```python
from build123d import *

# Parameters (mm, degrees)
F0_W      = 40
F0_H      = 20
F1_DEPTH  = 25
F2_W      = 10
F2_H      = 40
F3_DEPTH  = 25
F4_W      = 10
F4_H      = 2.6823076606
F5_DEPTH  = 50
F7_DEPTH  = 50
F8_R      = 14.99999
F9_F1_R   = 14.9999
F10_W     = 10
F10_H     = 10
F11_DEPTH = 100


# Not quite as in the source:
# - a fillet or chamfer is up to 0.001 mm smaller than in the source, because OpenCascade refuses the exact size


with BuildPart() as f1:
    # F0 (on Right) → F1 (new body)
    with BuildSketch(Plane.YZ):
        with Locations((20, 10)):
            Rectangle(F0_W, F0_H)
    extrude(amount=F1_DEPTH)

    # F2 (on face) → F3 (join)
    with BuildSketch(Plane.XY.offset(20)):
        with Locations((5, 20)):
            Rectangle(F2_W, F2_H)
    extrude(amount=F3_DEPTH)

    # F4 (on face) → F5 (cut)
    with BuildSketch(Plane.YZ.offset(10)):
        with BuildLine():
            Line((15, 45), (15, 35))
            ThreePointArc((15, 35), (20, 30), (25, 35))
            Line((25, 35), (25, 45))
            Line((25, 45), (15, 45))
        make_face()
        with Locations((20, 46.3411538303)):
            Rectangle(F4_W, F4_H)
    extrude(amount=-F5_DEPTH, mode=Mode.SUBTRACT)

    # F6 (on face) → F7 (cut)
    with BuildSketch(Plane.XY.offset(20)):
        with BuildLine():
            Line((25, 22.5), (15, 22.5))
            ThreePointArc((15, 22.5), (12.5, 20), (15, 17.5))
            Line((15, 17.5), (25, 17.5))
            Line((25, 17.5), (25, 22.5))
        make_face()
    extrude(amount=-F7_DEPTH, mode=Mode.SUBTRACT)

    # F8 (radius 15 in the source; OpenCascade refuses exactly that, so slightly less here)
    f8_edges = [f1.edges().sort_by_distance(p)[0] for p in [
        (5, 40, 45),
        (5, 0, 45),
    ]]
    fillet(f8_edges, radius=F8_R)

    # F9: fillet of radius 15 on 2 edges, made by hand

    # F9_f1 (radius 15 in the source; OpenCascade refuses exactly that, so slightly less here)
    f9_f1_edges = [f1.edges().sort_by_distance(p)[0] for p in [
        (25, 8.75, 20),
    ]]
    fillet(f9_f1_edges, radius=F9_F1_R)

    # F10 (on face) → F11 (cut)
    with BuildSketch(Plane(origin=(0, 40, 0), x_dir=(-1, 0, 0), z_dir=(0, 1, 0))):
        with Locations((-15, 5)):
            Rectangle(F10_W, F10_H)
    extrude(amount=-F11_DEPTH, mode=Mode.SUBTRACT)


solid = f1.part
```
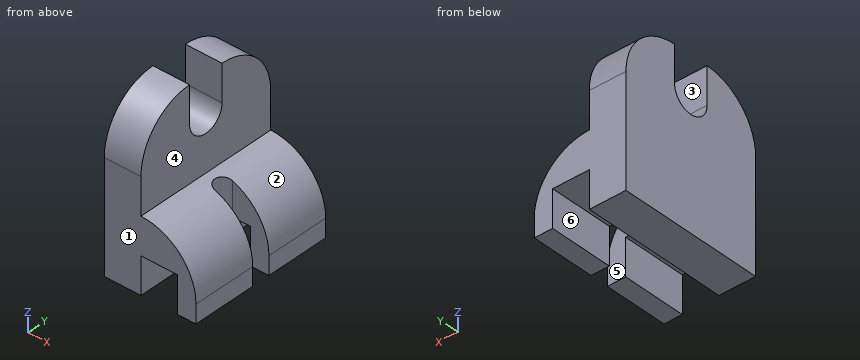
Source: CAD feature listing. Evaluate the final solid. Frame: model axes, mm. Face numbers are marked on the shaded views. A direction names the side the tool comes from. Coordinates: 2 decimals unless noted, no trailing zeros. Loops run counter-clockwise (first coordinate to the right, second up) from the corner with the lowest first, then second, coordinate; pieces in that order, holes last. Notation, with made-up numbers: (64, 0.25) -> (92, 0.25) arc R20 ccw to (92, 36.25) -> close; hole circle Ø6 at (37, 41.5). An arc over 180 degrees is marked (long way). One line per item, written item: value. Start each with the question number.
Q1. Line query: line 1 along X through (y, z) = (8, 5); line 2 along Y through (x, z) = (21.25, 4); line 3 along X through (y, z) = (22, 24.5). Output: solid intervals per line, ascending.
Q2. Contact query for flat-ended pins moving along their axis: P1, Ø6, axis at y = 21, z = 32.5, coming from the +X side; P2, Ø11, axis at x = 7, z = 38.5, coming from the +Y side; P3, Ø5, axis at x = 4.5, z = 40, coming from the -Y side. Output: stop coordinate, or through.
Q3. Section query C-C, the plane z = 18. Return the cut outline in (x, y).
Q4. Set-up query: the marked faces 4, 5 and 6. Return all of +Z, -Z, +X, -X, +Y, -Y with unobstructed straight access to the full face (end or side cutting, diameter ignored); none if empty.
Q5. Mould query, pull axis Y, two halves, no side actions, for the marked faces 1, 2 and 3. Classes: pulls with the +Y half, pulls with the -Y half, needs draft (parallel to the pull), parting line crosses it, or undercut.
Results:
1. line 1: 0 to 10, 20 to 25
1. line 2: 0 to 17.5, 22.5 to 40
1. line 3: 0 to 10
2. P1: x = 10
2. P2: y = 39.7
2. P3: y = 2.01
3. outline: (0, 0) -> (17.48, 0) -> (17.48, 17.5) -> (15, 17.5) arc R2.5 cw to (15, 22.5) -> (17.48, 22.5) -> (17.48, 40) -> (0, 40) -> close
4. face 4: +Z, +X, +Y, -Y
4. face 5: +Z, -Z, +X
4. face 6: -Z, +Y, -Y
5. face 1: pulls with the -Y half
5. face 2: needs draft
5. face 3: undercut
